Build history of the part. All positions in model axes, mm. Give positions to 0.01 mm unless a question says otherwise; leave off trailing zeros. Order: outer loops, then holes, each group sorted by start corner. A loop starts at its lowest first (then second) coordinate and runs counter-clockwise, first axis right, second up. Notation, with made-up numbers: (-3, 49) -> (21, 49) arc R25 cw to (21, 82) -> close; hole circle Ø2 at (40, 35). An arc over 180 degrees is marked (long way). One line per question, with ' | ' between items. Start each with the question number.
(1) Pin check, flat tips, straight feed: pin 1 Ø1.2 at (x, z) = (52, 1) entering from -Y; pin 2 Ø1.5 at (y, z) = (-43, 0.5) entering from +X; pin 3 Ø1.2 at (y, z) = (-18.5, 1) entering from +X; pin 4 Ø1.2 at (x, z) = (50, 1) entering from +Y. Stop position of each tip, or through.
(2) Cut at C-C (y = -22). Give the cut face in (x, z).
(3) Cut at B-B (x = -35.5). Give the cut face in (y, z).
(4) Cut at D-D (x = -14.5). Give the cut face in (y, z), then the cut area to 3 significant figures.
(5) Cut at A-A (y = -44). Give the cut face in (x, z).
(6) Drill centre lines: L1, parallel to Y at x = -2, z = 1.25; L2, parallel to X at y = -26.5, z = 1.2; L3, parallel to X at y = -92, z = 0.4. Where is each one in solid material? Low to high. Write a range as from..to.
from build123d import *

# Parameters (mm, degrees)
BOSS_EXTRUDE1_DEPTH = 2.5
FILLET1_R           = 2
FILLET2_R           = 10


with BuildPart() as part:
    # Sketch1 → Boss-Extrude1 (new body)
    with BuildSketch(Plane.XY):
        Polygon((-25.219628577, -20), (-32, -97.5), (-52.5, -97.5), (-52.5, -87.5), (-50, -87.5), (-50, -72.5), (-52.5, -72.5), (-52.5, -57.5), (-50, -57.5), (-50, -42.5), (-52.5, -42.5), (-52.5, -27.5), (-50, -27.5), (-50, -12.5), (-52.5, -12.5), (-52.5, 0), (-50, 0), (-45, 0), (-45, 2.5), (-37, 2.5), (-37, 0), (-24.5, 0), (-24.5, 2.5), (-16.5, 2.5), (-16.5, 0), (-4, 0), (-4, 2.5), (4, 2.5), (4, 0), (16.5, 0), (16.5, 2.5), (24.5, 2.5), (24.5, 0), (37, 0), (37, 2.5), (45, 2.5), (45, 0), (50, 0), (52.5, 0), (52.5, -12.5), (50, -12.5), (50, -27.5), (52.5, -27.5), (52.5, -42.5), (50, -42.5), (50, -57.5), (52.5, -57.5), (52.5, -72.5), (50, -72.5), (50, -87.5), (52.5, -87.5), (52.5, -97.5), (32, -97.5), (25.219628577, -20), align=None)
    extrude(amount=BOSS_EXTRUDE1_DEPTH)

    # Fillet1
    fillet1_edges = [part.edges().sort_by_distance(p)[0] for p in [
        (52.5, -97.5, 1.25),
        (32, -97.5, 1.25),
        (-32, -97.5, 1.25),
        (-52.5, -97.5, 1.25),
    ]]
    fillet(fillet1_edges, radius=FILLET1_R)

    # Fillet2
    fillet2_edges = [part.edges().sort_by_distance(p)[0] for p in [
        (25.219628577, -20, 1.25),
        (-25.219628577, -20, 1.25),
    ]]
    fillet(fillet2_edges, radius=FILLET2_R)


solid = part.part
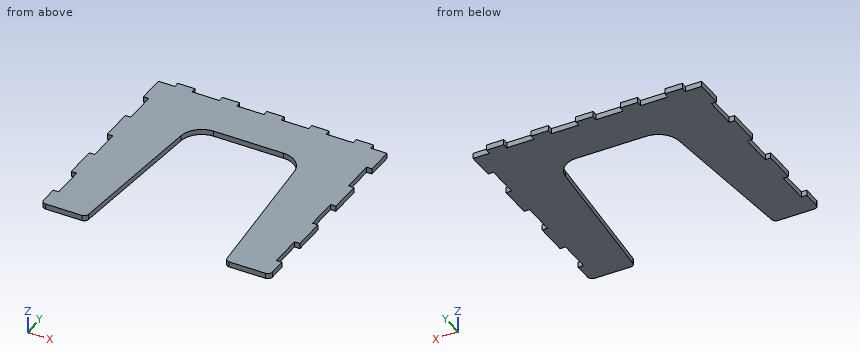
Result set:
1) pin 1: stops at y = -97.29 | pin 2: stops at x = 52.5 | pin 3: stops at x = 50 | pin 4: stops at y = 0
2) outline: (-50, 0) -> (-22.06, 0) -> (-22.06, 2.5) -> (-50, 2.5) -> close; (22.06, 0) -> (50, 0) -> (50, 2.5) -> (22.06, 2.5) -> close
3) outline: (-97.5, 0) -> (0, 0) -> (0, 2.5) -> (-97.5, 2.5) -> close
4) outline: (-20, 0) -> (0, 0) -> (0, 2.5) -> (-20, 2.5) -> close | area: 50.0 mm2
5) outline: (-50, 0) -> (-27.32, 0) -> (-27.32, 2.5) -> (-50, 2.5) -> close; (27.32, 0) -> (50, 0) -> (50, 2.5) -> (27.32, 2.5) -> close
6) L1: y = -20..2.5 | L2: x = -50..-25.42, 25.42..50 | L3: x = -52.5..-31.52, 31.52..52.5
